```python
from build123d import *

# Parameters (mm, degrees)
BOSS_EXTRUDE1_DEPTH = 25.4
BOSS_EXTRUDE2_REACH = 380.558
SKETCH2_W           = 50.8
SKETCH2_H           = 6.35
SKETCH3_W           = 25.4
SKETCH3_H           = 6.35
BOSS_EXTRUDE3_DEPTH = 6.35
SKETCH4_W           = 50.8
SKETCH4_H           = 6.35
BOSS_EXTRUDE4_DEPTH = 25.4


with BuildPart() as part:
    # Sketch1 → Boss-Extrude1 (new, symmetric)
    with BuildSketch(Plane(origin=(0, 0, 0), x_dir=(0, 0, -1), z_dir=(1, 0, 0))):
        with BuildLine():
            Line((-107.95, 0), (-107.95, -69.85))
            Line((-107.95, -69.85), (-101.6, -69.85))
            Line((-101.6, -69.85), (-101.6, 0))
            ThreePointArc((-101.6, 0), (0, 101.6), (101.6, 0))
            Line((101.6, 0), (101.6, -69.85))
            Line((101.6, -69.85), (107.95, -69.85))
            Line((107.95, -69.85), (107.95, 0))
            ThreePointArc((107.95, 0), (0, 107.95), (-107.95, 0))
        make_face()
    extrude(amount=BOSS_EXTRUDE1_DEPTH, both=True)

    # Sketch2 → Boss-Extrude2 (add, up to next)
    with BuildSketch(Plane.XY.offset(254), mode=Mode.PRIVATE) as boss_extrude2_sk1:
        with Locations((0, -66.675)):
            Rectangle(SKETCH2_W, SKETCH2_H)
    boss_extrude2_tool1 = extrude(boss_extrude2_sk1.sketch, amount=-BOSS_EXTRUDE2_REACH, mode=Mode.PRIVATE) - part.part
    boss_extrude2 = boss_extrude2_tool1.solids().sort_by_distance((0, -66.675, 254))[0]
    add(boss_extrude2)

    # Mirror1: Boss-Extrude2 across plane
    add(boss_extrude2.mirror(Plane.XY))

    # Sketch3 → Boss-Extrude3 (add)
    with BuildSketch(Plane(origin=(0, -63.5, 0), x_dir=(1, 0, 0), z_dir=(0, 1, 0))):
        with Locations((0, -257.175)):
            Rectangle(SKETCH3_W, SKETCH3_H)
    boss_extrude3 = extrude(amount=-BOSS_EXTRUDE3_DEPTH)

    # Mirror2: Boss-Extrude3 across plane
    add(boss_extrude3.mirror(Plane.XY))

    # Sketch4 → Boss-Extrude4 (add)
    with BuildSketch(Plane(origin=(0, -63.5, 0), x_dir=(1, 0, 0), z_dir=(0, 1, 0))):
        with Locations((0, -250.825)):
            Rectangle(SKETCH4_W, SKETCH4_H)
    boss_extrude4 = extrude(amount=BOSS_EXTRUDE4_DEPTH)

    # Mirror3: Boss-Extrude4 across plane
    add(boss_extrude4.mirror(Plane.XY))


solid = part.part
```
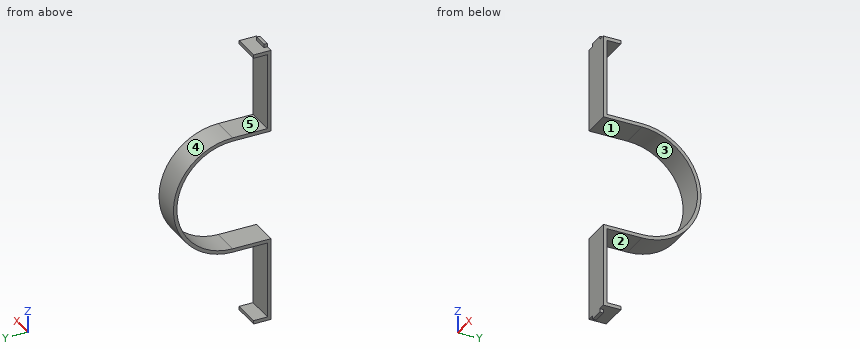
Geometry check sheet. Reference: the model listing, model coordinates, mm. Face numbers are marked on the shaded views. A direction names the side the tool comes from. Round coordinates to 2 decimals unless told otherwise and drop trailing zeros. Write each loop counter-clockwise with the first axis right and the second up, starting at its lowest first coordinate (ties: lowest second). Pieces come first, ordered by that corner, then holes. Notation, with made-up numbers: (-28.75, 72) -> (17.25, 72) arc R26 ccw to (17.25, 111) -> close; hole circle Ø3 at (54, -17.75). An arc over 180 degrees is marked (long way). Put each result on its own line as item: value.
1) Access from +Z, -Z, +X, -X, +Y, -Y to the whole of each face (thin tool, end or side, straight path). Record for the marked faces 1 and 2.
Recorded:
face 1: +X, -X, -Y
face 2: +X, -X, +Y
2) Cross-section at D-D, the plane z = 0. Enter the section's corners in (x, y).
Recorded:
outline: (-25.4, 101.6) -> (25.4, 101.6) -> (25.4, 107.95) -> (-25.4, 107.95) -> close
3) Depth check by flat-ended pin: P1, Ø3, axis at x = 20, y = 54, coming from the -Z side; P2, Ø9.5, axis at x = -12.5, y = -53.5, coming from the +Z side; P3, Ø3, axis at y = -67, z = -258.5, coming from the -X side. Enter the tip coordinate at first touch or a pass-through.
Recorded:
P1: stops at z = -94.32
P2: stops at z = 254
P3: stops at x = -12.7
4) Thickness scan on probe 1 along Z at (x, y) = (-6, -46); probe 2 along Y at (x, z) = (-3, 112); probe 3 along Z at (x, y) = (-10, 92). Record the ranges inside material, lowest first. Write a range as from..to.
Recorded:
probe 1: z = -254..-247.65, -107.95..-101.6, 101.6..107.95, 247.65..254
probe 2: y = -69.85..-63.5
probe 3: z = -56.47..-43.11, 43.11..56.47
5) Cross-section at A-A, the plane y = -43.5. Enter the section's corners in (x, z), plus the area to 3 significant figures.
Recorded:
outline: (-25.4, -254) -> (25.4, -254) -> (25.4, -247.65) -> (-25.4, -247.65) -> close; (-25.4, -107.95) -> (25.4, -107.95) -> (25.4, -101.6) -> (-25.4, -101.6) -> close; (-25.4, 101.6) -> (25.4, 101.6) -> (25.4, 107.95) -> (-25.4, 107.95) -> close; (-25.4, 247.65) -> (25.4, 247.65) -> (25.4, 254) -> (-25.4, 254) -> close
area: 1,290 mm2
6) Release check for a two-part mould opening along Z. For the marked faces 3, 4 and 5 record: pulls with the +Z half, pulls with the -Z half, needs draft (parallel to the pull), parting line crosses it, or undercut.
Recorded:
face 3: undercut
face 4: parting line crosses it
face 5: undercut
7) Cross-section at C-C, the plane y = 37.5. Enter the section's corners in (x, z).
Recorded:
outline: (-25.4, -101.23) -> (25.4, -101.23) -> (25.4, -94.43) -> (-25.4, -94.43) -> close; (-25.4, 94.43) -> (25.4, 94.43) -> (25.4, 101.23) -> (-25.4, 101.23) -> close
8) Cross-section at B-B, the plane x = -2.5. Enter the section's corners in (y, z), plus the area to 3 significant figures.
Recorded:
outline: (-69.85, -260.35) -> (-63.5, -260.35) -> (-63.5, -254) -> (-38.1, -254) -> (-38.1, -247.65) -> (-63.5, -247.65) -> (-63.5, -107.95) -> (0, -107.95) arc R107.95 ccw to (0, 107.95) -> (-63.5, 107.95) -> (-63.5, 247.65) -> (-38.1, 247.65) -> (-38.1, 254) -> (-63.5, 254) -> (-63.5, 260.35) -> (-69.85, 260.35) -> (-69.85, 101.6) -> (0, 101.6) arc R101.6 cw to (0, -101.6) -> (-69.85, -101.6) -> close
area: 5,240 mm2
